Drawing for the job (mm, zero at the part's lowest x, y, z). Coordinates: 2 decimals unless noted, no trailing zeros. Write each loop counter-clockwise with the first axis right and the second up, starting at its lowest first coordinate (ties: lowest second). Pieces come first, ordered by that corner, then holes. Notation, with made-up numbers: (58, -21.5) -> (93, -21.5) arc R16 ccw to (93, -17.5) -> close; hole circle Ø10 at (18.5, -19). An arc over 180 degrees is marked (long way). Write item = value, one per line. Start each with the question number.
Q1. Probe line 1 (Y direction, x = 12, z = 73.5); line 2 (Z direction, x = 45, y = 69); line 3 (X direction, y = 26, z = 45). List the from-to ranges inside material, lowest first.
Q2. Band-saw the part on B-B, the plane y = 44. List the corners of the cut face in (x, z).
Q3. Band-saw the part on A-A, the plane y = 80.5. List the corners of the cut face in (x, z), plus the area to 3 significant figures.
Q4. Pin check, flat tips, straight feed: P1, Ø10, axis at y = 16.5, z = 78.5, coming from the +X side; P2, Ø2, axis at x = 57.5, y = 18, coming from the +Z side; P3, Ø5, axis at y = 51, z = 36, coming from the -X side. Stop position of each tip, or through.
Q5. Pull direction X, two halves, no side cores. Call the marked faces 1, 2 and 3: released by +X, released by -X, zero draft, split by the parting line, or undercut.
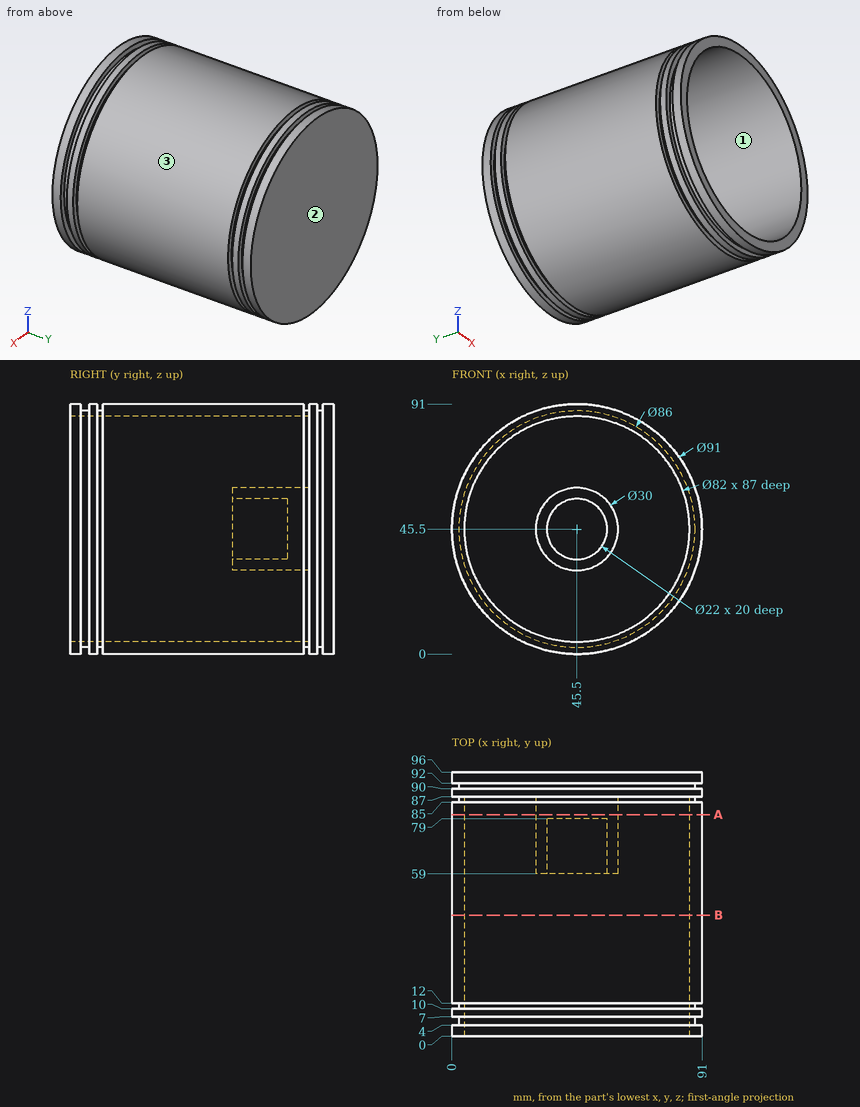
Ans:
q1.line_1 = 0 to 4, 7 to 10, 12 to 85, 87 to 90, 92 to 96
q1.line_2 = 0 to 4.5, 30.51 to 34.51, 56.49 to 60.49, 86.5 to 91
q1.line_3 = 0 to 4.5, 86.5 to 91
q2.outline = circle Ø91 at (45.5, 45.5); hole circle Ø82 at (45.5, 45.5)
q3.outline = circle Ø91 at (45.5, 45.5); circle Ø30 at (45.5, 45.5); hole circle Ø82 at (45.5, 45.5)
q3.area = 1,930 mm2
q4.P1 = 81.36
q4.P2 = 89.65
q4.P3 = 0.54
q5.face_1 = undercut
q5.face_2 = zero draft
q5.face_3 = split by the parting line
